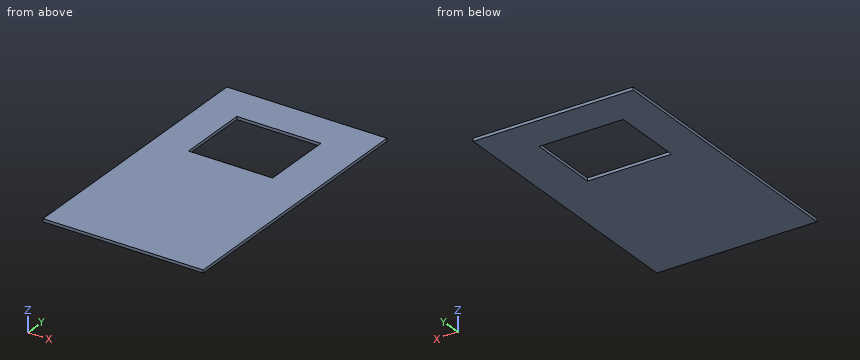
```python
from build123d import *

# Parameters (mm, degrees)
ESQUISSE1_W                  = 233
ESQUISSE1_H                  = 400
BOSS_EXTRU_1_DEPTH           = 4.2
ENL_V_MAT_EXTRU_1_DEPTH      = 279.375274783
ENL_V_MAT_EXTRU_1_DEPTH_BACK = 279.375274783
ESQUISSE2_W                  = 122.323690039
ESQUISSE2_H                  = 105.15953143


with BuildPart() as part:
    # Esquisse1 → Boss.-Extru.1 (new body)
    with BuildSketch(Plane.XY):
        with Locations((-45.332061069, -26.463104326)):
            Rectangle(ESQUISSE1_W, ESQUISSE1_H)
    extrude(amount=BOSS_EXTRU_1_DEPTH)

    # Esquisse2 → Enlèv. mat.-Extru.1 (cut, two sides: drawn at the far end of the back side and taken through both)
    with BuildSketch(Plane.XY.offset(4.2).offset(-ENL_V_MAT_EXTRU_1_DEPTH_BACK)):
        with Locations((-49.296189184, 65.859991666)):
            Rectangle(ESQUISSE2_W, ESQUISSE2_H)
    extrude(amount=ENL_V_MAT_EXTRU_1_DEPTH + ENL_V_MAT_EXTRU_1_DEPTH_BACK, mode=Mode.SUBTRACT)


solid = part.part
```
Check sheet for the modelled part. Datum: model origin and axes. Units: mm. Round coordinates to 2 decimals unless told otherwise and drop trailing zeros. Loops run counter-clockwise (first coordinate to the right, second up) from the corner with the lowest first, then second, coordinate; pieces in that order, holes last. Notation, with made-up numbers: (6, 85) - (26, 85) arc R30 cw to (26, 112) - close; hole circle Ø6 at (35, 55.25). An arc over 180 degrees is marked (long way). Write item = value, one per line. Start each with the question number.
Q1. Thickness scan on L1, parallel to Y at x = -109.5, z = 2.6. Record the ranges inside material, lowest first.
Q2. Section check B-B (z = 2.45). Record the boundary of the cut face in (x, y), plus the area to 3 significant figures.
Q3. Section check A-A (x = -22). Record the boundary of the cut face in (y, z), plus the area to 3 significant figures.
Q4. Section check C-C (y = 78.5). Record the boundary of the cut face in (x, z), plus the area to 3 significant figures.
Derived:
q1.L1 = -226.46 to 13.28, 118.44 to 173.54
q2.outline = (-161.83, -226.46) - (71.17, -226.46) - (71.17, 173.54) - (-161.83, 173.54) - close; hole (-110.46, 13.28) - (11.87, 13.28) - (11.87, 118.44) - (-110.46, 118.44) - close
q2.area = 80,300 mm^2
q3.outline = (-226.46, 0) - (13.28, 0) - (13.28, 4.2) - (-226.46, 4.2) - close; (118.44, 0) - (173.54, 0) - (173.54, 4.2) - (118.44, 4.2) - close
q3.area = 1,240 mm^2
q4.outline = (-161.83, 0) - (-110.46, 0) - (-110.46, 4.2) - (-161.83, 4.2) - close; (11.87, 0) - (71.17, 0) - (71.17, 4.2) - (11.87, 4.2) - close
q4.area = 465 mm^2
